Check sheet for the modelled part. Datum: model origin and axes. Units: mm. A direction names the side the tool comes from. Give positions to 0.01 mm unless a question says otherwise; leave off trailing zeros. Write each loop counter-clockwise with the first axis right and the second up, starting at its lowest first coordinate (ties: lowest second). Pieces come first, ordered by that corner, then holes. Notation, with made-up numbers: (3.5, 56) -> (20.5, 56) arc R17 ccw to (20.5, 84) -> close; hole circle Ø4 at (72, -4.5). An arc over 180 degrees is marked (long way). Return JSON: item names as keys, results as strings.
from build123d import *

# Parameters (mm, degrees)
SKETCH1_W           = 38.354
SKETCH1_H           = 38.2778
BOARD_DEPTH         = 1.2319
SKETCH3_W           = 25.146
SKETCH3_H           = 25.146
GPS_DEPTH           = 4.0767
SKETCH5_W           = 21.4376
SKETCH5_H           = 16.7894
UBLOCK_CHIP_DEPTH   = 2.4257
SKETCH6_R           = 3.3782
BATTERY_DEPTH       = 2.1082
SKETCH7_W           = 4.318
SKETCH7_H           = 7.9502
CONNECTOR_DEPTH     = 2.9972
SKETCH8_W           = 7.239
SKETCH8_H           = 2.286
CUT_EXTRUDE1_DEPTH  = 3.7592
CUT_EXTRUDE2_REACH  = 56.352
SKETCH9_R           = 1.6891
SKETCH10_R          = 1.8161
BOSS_EXTRUDE6_DEPTH = 0.1778


with BuildPart() as part:
    # Sketch1 → Board (new body)
    with BuildSketch(Plane(origin=(0, 0, 0), x_dir=(1, 0, 0), z_dir=(0, 1, 0))):
        with Locations((19.177, 19.1389)):
            Rectangle(SKETCH1_W, SKETCH1_H)
    extrude(amount=BOARD_DEPTH)

    # Sketch3 → GPS (add)
    with BuildSketch(Plane(origin=(0, 1.2319, 0), x_dir=(1, 0, 0), z_dir=(0, 1, 0))):
        with Locations((19.177, 19.1389)):
            Rectangle(SKETCH3_W, SKETCH3_H)
    extrude(amount=GPS_DEPTH)

    # Sketch5 → uBlock chip (add)
    with BuildSketch(Plane.XZ):
        with Locations((19.1008, -10.2108)):
            Rectangle(SKETCH5_W, SKETCH5_H)
    extrude(amount=UBLOCK_CHIP_DEPTH)

    # Sketch6 → Battery (add)
    with BuildSketch(Plane(origin=(0, 0, 0), x_dir=(-1, 0, 0), z_dir=(0, -1, 0))):
        with Locations(Location((-22.2758, 32.6263, 0), (0, 0, 90))):
            Circle(SKETCH6_R)
    extrude(amount=BATTERY_DEPTH)

    # Sketch7 → Connector (add)
    with BuildSketch(Plane(origin=(0, 0, 0), x_dir=(-1, 0, 0), z_dir=(0, -1, 0))):
        with Locations((-35.687, 27.3304)):
            Rectangle(SKETCH7_W, SKETCH7_H)
    extrude(amount=CONNECTOR_DEPTH)

    # Sketch8 → Cut-Extrude1 (cut)
    with BuildSketch(Plane(origin=(37.846, 0, 0), x_dir=(0, 0, -1), z_dir=(1, 0, 0))):
        with Locations((27.3304, -1.4986)):
            Rectangle(SKETCH8_W, SKETCH8_H)
    extrude(amount=-CUT_EXTRUDE1_DEPTH, mode=Mode.SUBTRACT)

    # Sketch9 → Cut-Extrude2 (cut, up to next)
    with BuildSketch(Plane(origin=(0, 1.2319, 0), x_dir=(1, 0, 0), z_dir=(0, 1, 0)), mode=Mode.PRIVATE) as cut_extrude2_sk1:
        with Locations(Location((34.9885, 3.3655, 0), (0, 0, 270))):
            Circle(SKETCH9_R)
    cut_extrude2_tool1 = extrude(cut_extrude2_sk1.sketch, amount=-CUT_EXTRUDE2_REACH, mode=Mode.PRIVATE) & part.part
    # Sketch9 → Cut-Extrude2 (cut, up to next)
    with BuildSketch(Plane(origin=(0, 1.2319, 0), x_dir=(1, 0, 0), z_dir=(0, 1, 0)), mode=Mode.PRIVATE) as cut_extrude2_sk2:
        with Locations(Location((3.3655, 3.3655, 0), (0, 0, 270))):
            Circle(SKETCH9_R)
    cut_extrude2_tool2 = extrude(cut_extrude2_sk2.sketch, amount=-CUT_EXTRUDE2_REACH, mode=Mode.PRIVATE) & part.part
    # Sketch9 → Cut-Extrude2 (cut, up to next)
    with BuildSketch(Plane(origin=(0, 1.2319, 0), x_dir=(1, 0, 0), z_dir=(0, 1, 0)), mode=Mode.PRIVATE) as cut_extrude2_sk3:
        with Locations(Location((3.3655, 34.9123, 0), (0, 0, 270))):
            Circle(SKETCH9_R)
    cut_extrude2_tool3 = extrude(cut_extrude2_sk3.sketch, amount=-CUT_EXTRUDE2_REACH, mode=Mode.PRIVATE) & part.part
    # Sketch9 → Cut-Extrude2 (cut, up to next)
    with BuildSketch(Plane(origin=(0, 1.2319, 0), x_dir=(1, 0, 0), z_dir=(0, 1, 0)), mode=Mode.PRIVATE) as cut_extrude2_sk4:
        with Locations(Location((34.9885, 34.9123, 0), (0, 0, 270))):
            Circle(SKETCH9_R)
    cut_extrude2_tool4 = extrude(cut_extrude2_sk4.sketch, amount=-CUT_EXTRUDE2_REACH, mode=Mode.PRIVATE) & part.part
    add(cut_extrude2_tool1.solids().sort_by_distance((34.9885, 1.2319, -3.3655))[0], mode=Mode.SUBTRACT)
    add(cut_extrude2_tool2.solids().sort_by_distance((3.3655, 1.2319, -3.3655))[0], mode=Mode.SUBTRACT)
    add(cut_extrude2_tool3.solids().sort_by_distance((3.3655, 1.2319, -34.9123))[0], mode=Mode.SUBTRACT)
    add(cut_extrude2_tool4.solids().sort_by_distance((34.9885, 1.2319, -34.9123))[0], mode=Mode.SUBTRACT)

    # Sketch10 → Boss-Extrude6 (add)
    with BuildSketch(Plane(origin=(0, 5.3086, 0), x_dir=(1, 0, 0), z_dir=(0, 1, 0))):
        with Locations(Location((17.5387, 20.7518, 0), (0, 0, 90))):
            Circle(SKETCH10_R)
    extrude(amount=BOSS_EXTRUDE6_DEPTH)


solid = part.part
(1) Cross-section at B-B on y = -1.25. Enter the section's corners in (x, z), then the cut area to 3 significant figures.
Reply:
{"outline": "(8.38, -18.61) -> (29.82, -18.61) -> (29.82, -1.82) -> (8.38, -1.82) -> close; circle Ø6.76 at (22.28, -32.63); (33.53, -31.31) -> (37.85, -31.31) -> (37.85, -30.95) -> (34.09, -30.95) -> (34.09, -23.71) -> (37.85, -23.71) -> (37.85, -23.36) -> (33.53, -23.36) -> close", "area": "403 mm^2"}
(2) Thickness scan on L1, parallel to X at y = 4, z = -13.5; L2, parallel to Y at x = 33, z = -32.5; L3, parallel to Y at x = 15.5, z = -14. Record the ranges inside material, lowest first.
Reply:
{"L1": "6.6 to 31.75", "L2": "0 to 1.23", "L3": "-2.43 to 5.31"}
(3) Set-up check for faces 1 (the flat face through (22, -2.108, -33)), 2 (the cylindrical face through (19.28, -1.04, -34.19)), 3 (the flat face through (29.82, -1, -10)): record each of +Z, -Z, +X, -X, +Y, -Y from which the full face is reachable in a straight line by a thin tool's end or side.
Reply:
{"face 1": "-Z, -X, -Y", "face 2": "-Y", "face 3": "+Z, -Z, +X, -Y"}
(4) Cross-section at A-A on z = -8.5. Enter the section's corners in (x, y), then the cut area to 3 significant figures.
Reply:
{"outline": "(0, 0) -> (8.38, 0) -> (8.38, -2.43) -> (29.82, -2.43) -> (29.82, 0) -> (38.35, 0) -> (38.35, 1.23) -> (31.75, 1.23) -> (31.75, 5.31) -> (6.6, 5.31) -> (6.6, 1.23) -> (0, 1.23) -> close", "area": "202 mm^2"}
(5) Release check for a two-part mould opening along X. For faces 4 (the flat face through (36, -2.642, -27)), 5 (the cylindrical face through (33.49, 0.62, -2.59)), 6 (the flat face through (8.382, -1, -10)) record: pulls with the +X half, pulls with the -X half, needs draft (parallel to the pull), parting line crosses it, or undercut.
Reply:
{"face 4": "needs draft", "face 5": "undercut", "face 6": "pulls with the -X half"}
(6) Cross-section at D-D on z = -4. Enter the section's corners in (x, y).
Reply:
{"outline": "(0, 0) -> (1.8, 0) -> (1.8, 1.23) -> (0, 1.23) -> close; (4.93, 0) -> (8.38, 0) -> (8.38, -2.43) -> (29.82, -2.43) -> (29.82, 0) -> (33.42, 0) -> (33.42, 1.23) -> (4.93, 1.23) -> close; (36.55, 0) -> (38.35, 0) -> (38.35, 1.23) -> (36.55, 1.23) -> close"}
(7) Cross-section at C-C on x = 36. Enter the section's corners in (y, z), then the cut area to 3 significant figures.
Reply:
{"outline": "(-3, -31.31) -> (0, -31.31) -> (0, -33.56) -> (1.23, -33.56) -> (1.23, -4.72) -> (0, -4.72) -> (0, -23.36) -> (-3, -23.36) -> close; (0, -38.28) -> (1.23, -38.28) -> (1.23, -36.27) -> (0, -36.27) -> close; (0, -2.01) -> (1.23, -2.01) -> (1.23, 0) -> (0, 0) -> close; hole (-2.64, -30.95) -> (-0.36, -30.95) -> (-0.36, -23.71) -> (-2.64, -23.71) -> close", "area": "47.8 mm^2"}
(8) Depth check by flat-ended pin: pin 1 Ø1.9 at (y, z) = (-1.5, -14) entering from -X; pin 2 Ø2 at (x, y) = (18, 3.5) entering from +Z; pin 3 Ø5 at (x, z) = (33, -7) entering from +Y. Enter the tip coordinate at first touch or a pass-through.
Reply:
{"pin 1": "x = 8.38", "pin 2": "z = -6.57", "pin 3": "y = 5.31"}
